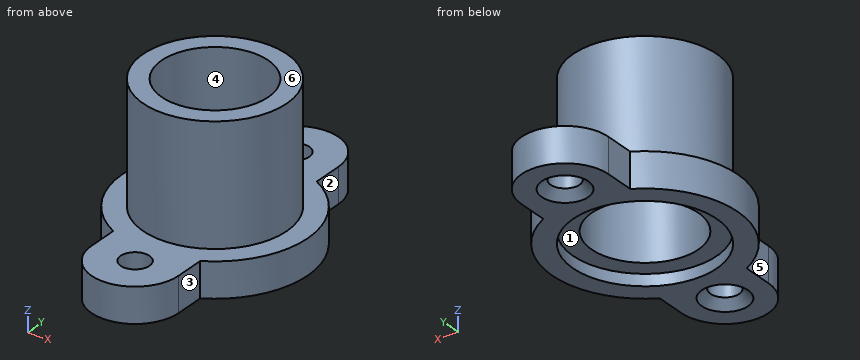
```python
from build123d import *

# Parameters (mm, degrees)
F2_R     = 2.5
F3_DEPTH = 6
F4_SIZE  = 1.5


with BuildPart() as f1:
    # F0 (on Front) → F1 (revolve)
    with BuildSketch(Plane.XZ):
        Polygon((12.4, 2), (12.4, 0), (16, 0), (16, 6), (12.4, 6), (12.4, 26.5), (9.2, 26.5), (9.2, 2), align=None)
    revolve(axis=Axis((0, 0, 0.530642), (0, 0, -1)))

    # F2 (on Top) → F3 (join)
    with BuildSketch(Plane.XY):
        with BuildLine():
            Line((7.5, 14.133294), (7.5, 19.4))
            ThreePointArc((7.5, 19.4), (0, 26.9), (-7.5, 19.4))
            Line((-7.5, 19.4), (-7.5, 14.133294))
            ThreePointArc((-7.5, 14.133294), (0, 16), (7.5, 14.133294))
        make_face()
        with Locations((0, 19.4)):
            Circle(F2_R, mode=Mode.SUBTRACT)
        with BuildLine():
            ThreePointArc((7.5, -14.133294), (0, -16), (-7.5, -14.133294))
            Line((-7.5, -14.133294), (-7.5, -19.4))
            ThreePointArc((-7.5, -19.4), (0, -26.9), (7.5, -19.4))
            Line((7.5, -19.4), (7.5, -14.133294))
        make_face()
        with Locations((0, -19.4)):
            Circle(F2_R, mode=Mode.SUBTRACT)
    extrude(amount=F3_DEPTH)

    # F4
    f4_edges = [f1.edges().sort_by_distance(p)[0] for p in [
        (-2.5, 19.4, 0),
        (-2.5, -19.4, 0),
    ]]
    chamfer(f4_edges, length=F4_SIZE)


solid = f1.part
```
Could you check a few things on this model? Use its own coordinates, in mm. Face numbers are marked on the shaded views. A direction names the side the tool comes from. Coordinates: 2 decimals unless noted, no trailing zeros. Loops run counter-clockwise (first coordinate to the right, second up) from the corner with the lowest first, then second, coordinate; pieces in that order, holes last. Notation, with made-up numbers: M 45,-18 L 75,-18 A31 cw 75,10 Z; hole C 75.25,72.5 d8. An arc over 180 degrees is marked long. Put each result on its own line as item: value. Start each with the question number.
(1) Suppose I cut it at C-C on z = 5. Please give me the cut outline in (x, y).
(2) Suppose I cut it at B-B on x = 0. Please give me the cut outline in (y, z), then the cut area to 3 significant figures.
(3) For the marked faces 1, 2 and 3, which set-ups out of +Z, -Z, +X, -X, +Y, -Y let a thin tool reach every point of the face, with its end or its side?
(4) Suppose I cut it at A-A on y = 0. Please give me the cut outline in (x, z), then the cut area to 3 significant figures.
(5) Suppose I cut it at D-D on z = 17.25. Please give me the cut outline in (x, y).
(6) Thinking about a two-plate mould opening in X: for the marked faces 4, 5 and 6, which applies, pulls with the +X half, pulls with the -X half, needs draft (parallel to the pull), parting line crosses it, or undercut?
(7) I need wall thicknesses on line 1 (Y direction, x = 0, z = 3.2); line 2 (X direction, y = 0, z = 0.55); line 3 (X direction, y = 0, z = 11.75). Which ranges of each line are inside material? Lowest first, please. Write a range as from..to.
(8) Will these pins go through, and if not, where does the flat tip stop? P1, Ø6, axis at x = 0, y = 19.4, coming from the +Z side; P2, Ø12, axis at x = 3.5, y = -15, coming from the -Z side; P3, Ø6, axis at x = -3.5, y = 0.5, coming from the -Z side; P4, Ø1.5, axis at x = -2, y = -17.5, coming from the -Z side.
Solutions:
1. outline: M -7.5,-19.4 A7.5 ccw 7.5,-19.4 L 7.5,-14.13 A16 ccw 7.5,14.13 L 7.5,19.4 A7.5 ccw -7.5,19.4 L -7.5,14.13 A16 ccw -7.5,-14.13 Z; hole C 0,0 d18.4; hole C 0,-19.4 d5; hole C 0,19.4 d5
2. outline: M -26.9,0 L -23.4,0 L -21.9,1.5 L -21.9,6 L -26.9,6 Z; M -16.9,1.5 L -15.4,0 L -12.4,0 L -12.4,2 L -9.2,2 L -9.2,26.5 L -12.4,26.5 L -12.4,6 L -16.9,6 Z; M 9.2,2 L 12.4,2 L 12.4,0 L 15.4,0 L 16.9,1.5 L 16.9,6 L 12.4,6 L 12.4,26.5 L 9.2,26.5 Z; M 21.9,1.5 L 23.4,0 L 26.9,0 L 26.9,6 L 21.9,6 Z
2. area: 266 mm2
3. face 1: -Z
3. face 2: +Z, -Z, +X, +Y
3. face 3: +Z, -Z, +X, -Y
4. outline: M -16,0 L -12.4,0 L -12.4,2 L -9.2,2 L -9.2,26.5 L -12.4,26.5 L -12.4,6 L -16,6 Z; M 9.2,2 L 12.4,2 L 12.4,0 L 16,0 L 16,6 L 12.4,6 L 12.4,26.5 L 9.2,26.5 Z
4. area: 200 mm2
5. outline: C 0,0 d24.8; hole C 0,0 d18.4
6. face 4: undercut
6. face 5: pulls with the -X half
6. face 6: needs draft
7. line 1: y = -26.9..-21.9, -16.9..-9.2, 9.2..16.9, 21.9..26.9
7. line 2: x = -16..-12.4, 12.4..16
7. line 3: x = -12.4..-9.2, 9.2..12.4
8. P1: stops at z = 6
8. P2: stops at z = 0
8. P3: passes through
8. P4: stops at z = 0.49
